Check sheet for the modelled part. Datum: model origin and axes. Units: mm. Face numbers are marked on the shaded views. A direction names the side the tool comes from. Coordinates: 2 decimals unless noted, no trailing zeros. Loops run counter-clockwise (first coordinate to the right, second up) from the corner with the lowest first, then second, coordinate; pieces in that order, holes last.
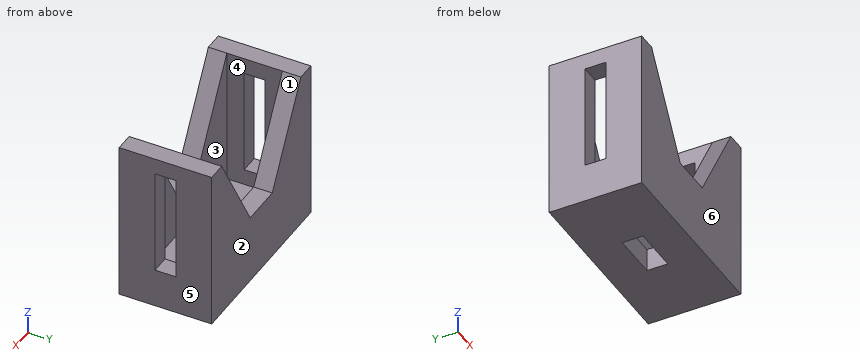
Autodesk Inventor part; units mm, degrees
ref_plane "YZ Plane" through (0, 0, 0) normal (1, 0, 0) x (0, 1, 0)
ref_plane "XZ Plane" through (0, 0, 0) normal (0, 1, 0) x (-1, 0, 0)
ref_plane "XY Plane" through (0, 0, 0) normal (0, 0, 1) x (1, 0, 0)
sketch "Náčrt1" plane through (0, 0, 0) normal (0, 0, 1) x (1, 0, 0)
  line L0 (0, 14) -> (0, -14)
  line L1 (-28, 0) -> (28, 0)
  line L2 (20, -10) -> (-20, -10)
  line L3 (-20, -10) -> (-20, 10)
  line L4 (-20, 10) -> (20, 10)
  line L5 (20, 10) -> (20, -10)
  point P0 (0, 0)
  dimension "d0" = 40
  dimension "d1" = 20
extrude "Vysunutí1" add sketch "Náčrt1" along normal blind 35
sketch "Náčrt2" plane through (0, 0, 35) normal (0, 0, 1) x (1, 0, 0)
  line L0 (20, 10) -> (-20, 10)
  line L1 (-20, 10) -> (-20, -10)
  line L2 (-20, -10) -> (20, -10)
  line L3 (20, -10) -> (20, 10)
  line L4 (-16, 6) -> (16, 6)
  line L5 (16, 6) -> (16, -6)
  line L6 (16, -6) -> (-16, -6)
  line L7 (-16, -6) -> (-16, 6)
  point P0 (0, 0)
  dimension "d4" = 4
extrude "Vysunutí2" cut sketch "Náčrt2" against normal blind 30 contours L4 L5 L6 L7
sketch "Náčrt3" plane through (0, 0, 5) normal (0, 0, 1) x (1, 0, 0)
  line L0 (16, -6) -> (-16, -6)
  line L1 (16, 6) -> (16, -6)
  line L2 (-16, 6) -> (16, 6)
  line L3 (-16, -6) -> (-16, 6)
  line L4 (0, 14) -> (0, -14)
  line L5 (-28, 0) -> (28, 0)
  line L6 (-5, 2.25) -> (5, 2.25)
  line L7 (5, 2.25) -> (5, -2.25)
  line L8 (5, -2.25) -> (-5, -2.25)
  line L9 (-5, -2.25) -> (-5, 2.25)
  point P0 (0, 0)
  dimension "d7" = 10
  dimension "d8" = 4.5
extrude "Vysunutí3" cut sketch "Náčrt3" against normal through all contours L8 L9 L5 L4 | L4 L5 L7 L8 | L5 L4 L6 L7 | L5 L9 L6 L4
sketch "Náčrt4" plane through (20, -10, 0) normal (1, 0, 0) x (0, 0, -1)
  line L0 (0, 0) -> (0, 20)
  line L1 (0, 20) -> (-35, 20)
  line L2 (-35, 0) -> (-35, 20)
  line L3 (0, 0) -> (-35, 0)
  line L4 (-42, 10) -> (7, 10)
  line L5 (0, -6) -> (0, 36)
  line L6 (-35, 16) -> (-5, 16)
  line L7 (-35, 4) -> (-5, 4)
  line L8 (-5, 16) -> (-5, 4)
  line L9 (-31.5, 7.75) -> (-8.5, 7.75)
  line L10 (-8.5, 7.75) -> (-8.5, 12.25)
  line L11 (-8.5, 12.25) -> (-31.5, 12.25)
  line L12 (-31.5, 12.25) -> (-31.5, 7.75)
  line L13 (-31.5, 10) -> (-8.5, 10)
  line L14 (-8.5, 10) -> (-8.5, 7.75)
  line L15 (-8.5, 7.75) -> (-31.5, 7.75)
  line L16 (-31.5, 7.75) -> (-31.5, 10)
  point P0 (0, 10)
  dimension "d11" = 4.5
  dimension "d12" = 23
  dimension "d13" = 3.5
extrude "Vysunutí4" cut sketch "Náčrt4" against normal through all contours L10 L9 L12 L4 | L4 L12 L11 L10
sketch "Náčrt5" plane through (-20, -10, 0) normal (0, -1, 0) x (1, 0, 0)
  line L0 (0, 0) -> (40, 0)
  line L1 (40, 0) -> (40, 35)
  line L2 (0, 35) -> (40, 35)
  line L3 (0, 0) -> (0, 35)
  line L4 (20, 42) -> (20, -7)
  line L5 (-8, 0) -> (48, 0)
  line L6 (4, 35) -> (4, 5)
  line L7 (36, 35) -> (36, 5)
  line L8 (4, 35) -> (15.547, 15)
  line L9 (24.453, 15) -> (36, 35)
  line L10 (24.453, 15) -> (15.547, 15)
  line L11 (36, 5) -> (4, 5)
  line L12 (4, 35) -> (36, 35)
  point P0 (20, 0)
  dimension "d16" = 30
  dimension "d17" = 30
  dimension "d18" = 10
extrude "Vysunutí5" cut sketch "Náčrt5" against normal through all contours L2 L4 L10 L8 | L4 L2 L9 L10
properties part number "uhelnik_30x30_M4_3D tisk"
(1) Section check B-B, the plane z = 13.5. Enter the section's corners in (x, y), plus the area to 3 significant figures.
(2) Set-up check for the marked faces 1, 2 and 3: record each of +Z, -Z, +X, -X, +Y, -Y from which the full face is reachable in a straight line by a thin tool's end or side.
(3) Section check C-C, the plane x = -1. Enter the section's corners in (y, z).
(4) Section check A-A, the plane y = -0.25. Enter the section's corners in (x, z).
(5) Section check D-D, the plane z = 5.5. Enter the section's corners in (x, y), plus the area to 3 significant figures.
(6) Scan lines: line 1 along Y through (x, z) = (-11, 10); line 2 along Y through (x, z) = (2, 2); line 3 along X through (y, z) = (-3.25, 12.5). Record each from-to range of solid material in increasing order.
(7) Gauge pin test, flat end, axial feed: P1, Ø1.2, axis at x = -1, y = -8, coming from the +Z side. Record the tip position at first contact, or that the pin passes through.
(8) Draft check along X on the marked faces 4, 5 and 6. Enter one of: pulls with the +X half, pulls with the -X half, needs draft (parallel to the pull), parting line crosses it, or undercut.
Determined:
1. outline: (-20, -10) - (20, -10) - (20, -2.25) - (16, -2.25) - (16, -6) - (-16, -6) - (-16, -2.25) - (-20, -2.25) - close; (-20, 2.25) - (-16, 2.25) - (-16, 6) - (16, 6) - (16, 2.25) - (20, 2.25) - (20, 10) - (-20, 10) - close
1. area: 380 mm2
2. face 1: +Z, +Y, -Y
2. face 2: +Z, -Z, +X, -X, +Y
2. face 3: +Z
3. outline: (-10, 0) - (-2.25, 0) - (-2.25, 5) - (-6, 5) - (-6, 15) - (-10, 15) - close; (2.25, 0) - (10, 0) - (10, 15) - (6, 15) - (6, 5) - (2.25, 5) - close
4. outline: (-20, 0) - (-5, 0) - (-5, 5) - (-16, 5) - (-16, 8.5) - (-20, 8.5) - close; (-20, 31.5) - (-16, 31.5) - (-16, 35) - (-20, 35) - close; (5, 0) - (20, 0) - (20, 8.5) - (16, 8.5) - (16, 5) - (5, 5) - close; (16, 31.5) - (20, 31.5) - (20, 35) - (16, 35) - close
5. outline: (-20, -10) - (20, -10) - (20, 10) - (-20, 10) - close; hole (-16, -6) - (16, -6) - (16, 6) - (-16, 6) - close
5. area: 416 mm2
6. line 1: y = -10 to -6, 6 to 10
6. line 2: y = -10 to -2.25, 2.25 to 10
6. line 3: x = -20 to -16, 16 to 20
7. P1: stops at z = 15
8. face 4: undercut
8. face 5: pulls with the +X half
8. face 6: needs draft
